Verification items for the finished model (mm, model axes). Face numbers are marked on the shaded views. Coordinates: 2 decimals unless noted, no trailing zeros. Write each loop counter-clockwise with the first axis right and the second up, starting at its lowest first coordinate (ties: lowest second). Pieces come first, ordered by that corner, then holes. Notation, with made-up numbers: M 23.5,5.25 L 41.5,5.25 A23 ccw 41.5,41.25 Z; hole C -0.5,44.5 d10. An arc over 180 degrees is marked long. Answer in a Markdown table with one row per item.
Autodesk Inventor part; units mm, degrees
ref_plane "YZ Plane" through (0, 0, 0) normal (1, 0, 0) x (0, 1, 0)
ref_plane "XZ Plane" through (0, 0, 0) normal (0, 1, 0) x (-1, 0, 0)
ref_plane "XY Plane" through (0, 0, 0) normal (0, 0, 1) x (1, 0, 0)
sketch "Sketch1" plane through (0, 0, 0) normal (0, 0, 1) x (1, 0, 0)
  line L0 (7.3323, 0) -> (3.6662, -6.35)
  line L1 (3.6662, -6.35) -> (-3.6662, -6.35)
  line L2 (-3.6662, -6.35) -> (-7.3323, 0)
  line L3 (-7.3323, 0) -> (-3.6662, 6.35)
  line L4 (-3.6662, 6.35) -> (3.6662, 6.35)
  line L5 (3.6662, 6.35) -> (7.3323, 0)
  point P0 (0, 0)
  point P1 (0, 0)
  dimension "d0" = 12.7
extrude "Extrusion1" add sketch "Sketch1" along normal mid plane 114.3
sketch "Sketch10" plane through (0, 0, -57.15) normal (0, 0, -1) x (-1, 0, 0)
  point P0 (0, 0)
  point P1 (0, 0)
hole "Hole3" at (0, 0, -57.15) direction (0, 0, 1) diameter 3.9624 depth 13.6144 tip angle 118
ref_plane "Work Plane4" through (0, 0, -46.99) normal (0, 0, -1) x (-1, 0, 0)
ref_plane "Work Plane5" through (0, 0, -8.636) normal (0, 0, -1) x (-1, 0, 0)
ref_plane "Work Plane6" through (0, 0, 18.2372) normal (0, 0, -1) x (-1, 0, 0)
sketch "Sketch13" plane through (0, 0, 18.2372) normal (0, 0, -1) x (-1, 0, 0)
  circle A0 centre (0, 0) radius 1.9812
  circle A1 centre (0, 0) radius 4.9784
  line L0 (3.6662, -6.35) -> (7.3323, 0)
  circle A2 centre (0, 0) radius 7.3323
  dimension "d51" = 9.9568
extrude "Extrusion7" cut sketch "Sketch13" against normal blind 1.0668 contours A2 L0 | L0 A2
ref_plane "Work Plane7" through (0, 0, 40.132) normal (0, 0, 1) x (1, 0, 0)
sketch "Sketch15" plane through (0, 0, 40.132) normal (0, 0, 1) x (1, 0, 0)
  circle A0 centre (0, 0) radius 1.9812
  circle A1 centre (0, 0) radius 4.9784
  line L0 (3.6662, -6.35) -> (7.3323, 0)
  circle A2 centre (0, 0) radius 7.3323
  dimension "d60" = 9.9568
extrude "Extrusion9" cut sketch "Sketch15" against normal blind 1.0668 contours A2 L0 | L0 A2
sketch "Sketch16" plane through (0, 0, 39.0652) normal (0, 0, 1) x (1, 0, 0)
  point P0 (0, 0)
sketch "Sketch17" plane through (0, 0, -46.99) normal (0, 0, -1) x (-1, 0, 0)
  circle A0 centre (0, 0) radius 1.9812
  circle A1 centre (0, 0) radius 5.5563
  line L0 (-3.6662, 6.35) -> (3.6662, 6.35)
  line L1 (3.6662, 6.35) -> (7.3323, 0)
  line L2 (7.3323, 0) -> (3.6662, -6.35)
  line L3 (3.6662, -6.35) -> (-3.6662, -6.35)
  line L4 (-3.6662, -6.35) -> (-7.3323, 0)
  line L5 (-7.3323, 0) -> (-3.6662, 6.35)
  dimension "d64" = 11.1125
extrude "Extrusion10" cut sketch "Sketch17" along normal blind 2.3368 and the other way blind 6.477 contours L0 L1 L2 L3 L4 L5
sketch "Sketch18" plane through (0, 0, -8.636) normal (0, 0, -1) x (-1, 0, 0)
  circle A0 centre (0, 0) radius 1.9812
  circle A1 centre (0, 0) radius 4.9784
  line L0 (3.6662, -6.35) -> (7.3323, 0)
  circle A2 centre (0, 0) radius 7.3323
  dimension "d69" = 9.9568
extrude "Extrusion11" cut sketch "Sketch18" against normal blind 1.0668 contours A2 L0 | L0 A2
properties part number "Ch-1-01-0.5x4.5HexShaft" material "Steel, Alloy"
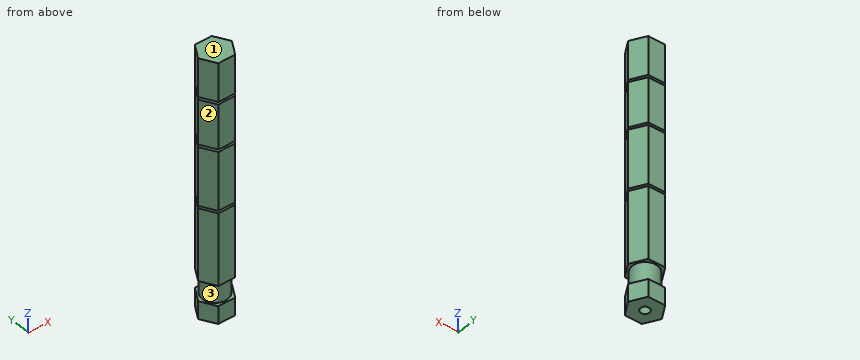
1) Depth check by flat-ended pin: pin 1 (3 mm diameter, centred on y = -4.5, z = 41, fed in from -X); pin 2 (3 mm diameter, centred on y = -3, z = -17.5, fed in from +X). Enter the tip coordinate at first touch or a pass-through.
Response values:
| item | result |
|---|---|
| pin 1 | stops at x = -5.6 |
| pin 2 | stops at x = 6.47 |
2) Sectioned sample at A-A (z = -27). Record the cut outline in (x, y).
Response values:
| item | result |
|---|---|
| outline | M -7.33,0 L -3.67,-6.35 L 3.67,-6.35 L 7.33,0 L 3.67,6.35 L -3.67,6.35 Z |
3) Release check for a two-part mould opening along Z. For the marked faces 1, 2 and 3 record: +Z half, -Z half, draft (parallel to the pull), parting line (faces both ways), or undercut.
Response values:
| item | result |
|---|---|
| face 1 | +Z half |
| face 2 | draft |
| face 3 | undercut |
4) Thickness scan on L1, parallel to Z at x = -6, y = 1.5; L2, parallel to Y at x = 0, z = -52; L3, parallel to X at y = 0, z = -51.5. Record the ranges inside material, lowest first. Write a range as [from, to].
Response values:
| item | result |
|---|---|
| L1 | z = [-57.15, -49.33], [-40.51, -8.64], [-7.57, 18.24], [19.3, 39.07], [40.13, 57.15] |
| L2 | y = [-6.35, -1.98], [1.98, 6.35] |
| L3 | x = [-7.33, -1.98], [1.98, 7.33] |
